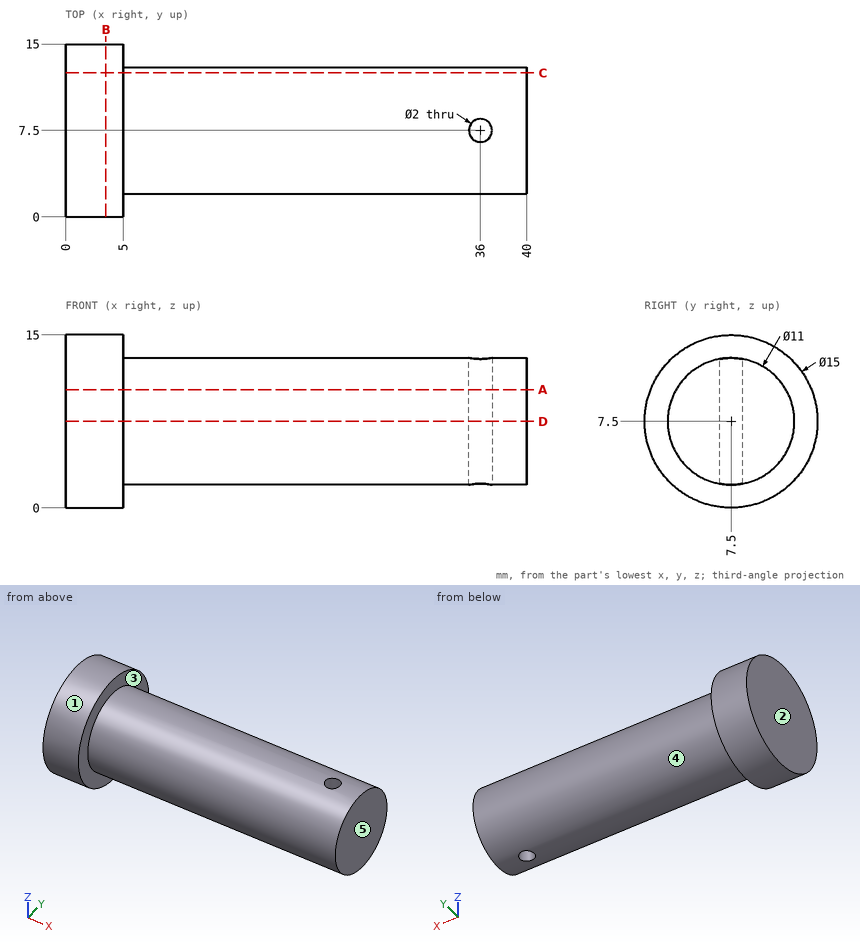
Drawing for the job (mm, zero at the part's lowest x, y, z). A direction names the side the tool comes from. Give positions to 0.01 mm unless a question says otherwise; leave off trailing zeros. Order: outer loops, then holes, each group sorted by start corner. A loop starts at its lowest first (then second) coordinate and runs counter-clockwise, first axis right, second up. Notation, with made-up numbers: (54.5, -33.75) - (60.5, -33.75) arc R21 ccw to (60.5, 3.25) - close; hole circle Ø5 at (75.25, 76). An arc over 180 degrees is marked (long way). Write item = value, one per line. Start each with the question number.
1. Two-plate mould, pull along X, no slides. Class the marked faces 1, 2 and 3: pulls with the +X half, pulls with the -X half, needs draft (parallel to the pull), parting line crosses it, or undercut.
2. Cut at C-C, the plane y = 12.5. List the corners of the cut face in (x, z).
3. Cut at B-B, the plane x = 3.5. List the corners of the cut face in (y, z), and give its area (3 significant figures).
4. Drop flat-ended pins along their axis: P1, Ø1, axis at x = 27, y = 3.5, coming from the -Z side; P2, Ø3, axis at x = 36, y = 7.5, coming from the -Z side; P3, Ø4, axis at x = 18, y = 10.5, coming from the -Z side. Give the stop position or say it passes through.
5. Cut at D-D, the plane z = 7.5. List the corners of the cut face in (x, y).
6. Which spindle directions (+Z, -Z, +X, -X, +Y, -Y) get a long thin tool onto all of the face, cutting with end or side? Do the marked faces 4 and 5. Say none if no direction does.
7. Probe line 1 along X through (y, z) = (7.5, 10); line 2 along Y through (x, z) = (36, 7.75); line 3 along Y through (x, z) = (36.5, 6). List the from-to ranges inside material, lowest first.
8. Cut at A-A, the plane z = 10.25. List the corners of the cut face in (x, y), and give its area (3 significant figures).
Taken from the geometry:
q1.face_1 = needs draft
q1.face_2 = pulls with the -X half
q1.face_3 = pulls with the +X half
q2.outline = (0, 1.91) - (5, 1.91) - (5, 5.21) - (40, 5.21) - (40, 9.79) - (5, 9.79) - (5, 13.09) - (0, 13.09) - close
q3.outline = circle Ø15 at (7.5, 7.5)
q3.area = 177 mm²
q4.P1 = 3.26
q4.P2 = 2
q4.P3 = 2.09
q5.outline = (0, 0) - (5, 0) - (5, 2) - (40, 2) - (40, 13) - (5, 13) - (5, 15) - (0, 15) - close; hole circle Ø2 at (36, 7.5)
q6.face_4 = +X
q6.face_5 = +Z, -Z, +X, +Y, -Y
q7.line_1 = 0 to 35, 37 to 40
q7.line_2 = 2.01 to 6.5, 8.5 to 12.99
q7.line_3 = 2.21 to 6.63, 8.37 to 12.79
q8.outline = (0, 0.52) - (5, 0.52) - (5, 2.74) - (40, 2.74) - (40, 12.26) - (5, 12.26) - (5, 14.48) - (0, 14.48) - close; hole circle Ø2 at (36, 7.5)
q8.area = 400 mm²
